For this review, use the dimensioned drawing (mm, ordinates from the lowest corner) and the shaded views. Coordinates: 2 decimals unless noted, no trailing zeros. Loops run counter-clockwise (first coordinate to the right, second up) from the corner with the lowest first, then second, coordinate; pieces in that order, holes last. Notation, with made-up numbers: M 14.5,7 L 67.5,7 A17 ccw 67.5,19 Z; hole C 25.5,75 d6. An arc over 180 degrees is marked long. One line per item, written item: value.
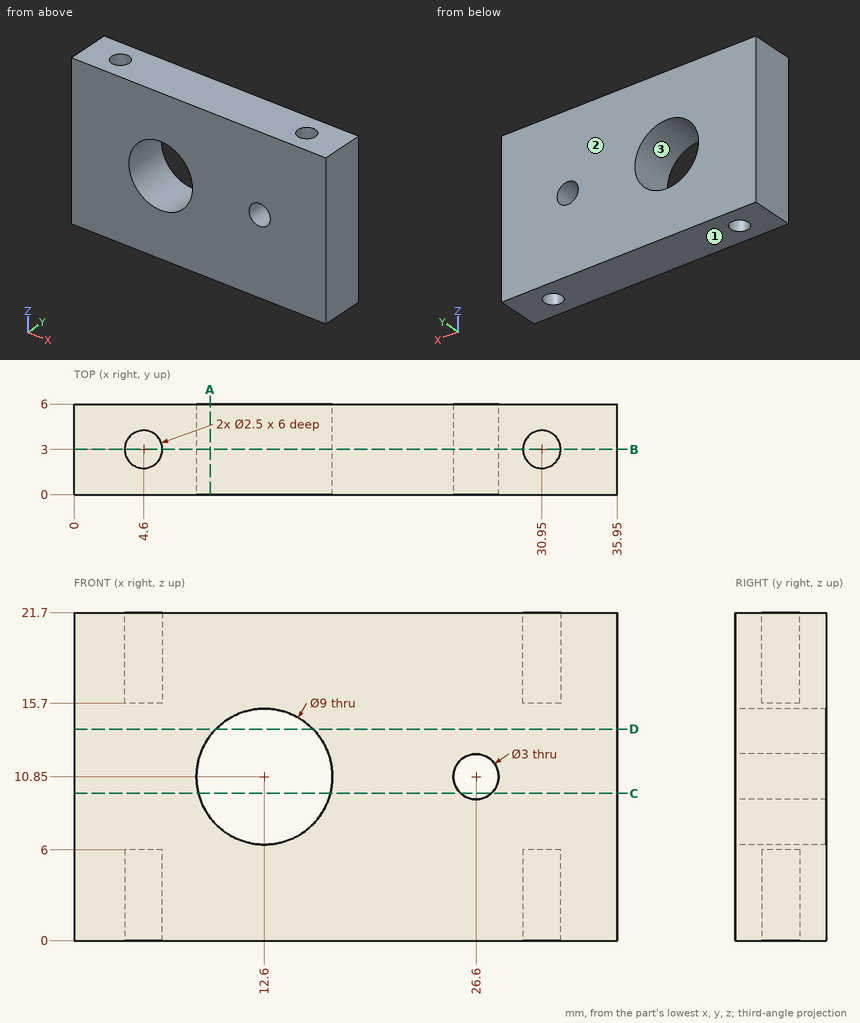
(1) Add section B-B on y = 3. State the section outline as (x, z) points.
Checks:
outline: M 0,0 L 3.35,0 L 3.35,6 L 5.85,6 L 5.85,0 L 29.7,0 L 29.7,6 L 32.2,6 L 32.2,0 L 35.95,0 L 35.95,21.7 L 32.2,21.7 L 32.2,15.7 L 29.7,15.7 L 29.7,21.7 L 5.85,21.7 L 5.85,15.7 L 3.35,15.7 L 3.35,21.7 L 0,21.7 Z; hole C 12.6,10.85 d9; hole C 26.6,10.85 d3
(2) Draft analysis for pull direction Z (two halves, no side actions). For the marked faces 1, 2 and 3, state which applies: pulls with the +Z half, pulls with the -Z half, needs draft (parallel to the pull), parting line crosses it, or undercut.
Checks:
face 1: pulls with the -Z half
face 2: needs draft
face 3: undercut
(3) Add section D-D on z = 14. State the section outline as (x, y) points, then the cut area to 3 significant figures.
Checks:
outline: M 0,0 L 9.39,0 L 9.39,6 L 0,6 Z; M 15.81,0 L 35.95,0 L 35.95,6 L 15.81,6 Z
area: 177 mm^2
(4) Add section C-C on z = 9.75. State the section outline as (x, y) points, then the cut area to 3 significant figures.
Checks:
outline: M 0,0 L 8.24,0 L 8.24,6 L 0,6 Z; M 16.96,0 L 25.58,0 L 25.58,6 L 16.96,6 Z; M 27.62,0 L 35.95,0 L 35.95,6 L 27.62,6 Z
area: 151 mm^2
(5) Insertion check: pin 1 Ø0.8 at (x, y) = (5, 3) entering from +Z; pin 2 Ø2 at (x, y) = (4.6, 3) entering from -Z; pin 3 Ø7 at (x, z) = (12.6, 10.85) entering from -Y. Each pin has a flat end and moves straight along its axis. Give the tip position at first contact, or say it passes through.
Checks:
pin 1: z = 15.7
pin 2: z = 6
pin 3: through
(6) To check wall thickness, follow L1, parallel to X at y = 3, z = 18.5; L2, parallel to X at y = 3.1, z = 10.85; L3, parallel to Y at x = 30.95, z = 19.15. State the ranges of each line that lie inside material, in increasing order. Write a range as [from, to].
Checks:
L1: [0, 3.35], [5.85, 29.7], [32.2, 35.95]
L2: [0, 8.1], [17.1, 25.1], [28.1, 35.95]
L3: [0, 1.75], [4.25, 6]
(7) Add section A-A on x = 9. State the section outline as (y, z) points.
Checks:
outline: M 0,0 L 6,0 L 6,8.15 L 0,8.15 Z; M 0,13.55 L 6,13.55 L 6,21.7 L 0,21.7 Z
